```python
from build123d import *

# Parameters (mm, degrees)
SKETCH1_R           = 3
BOSS_EXTRUDE1_DEPTH = 6.35


with BuildPart() as part:
    # Sketch1 → Boss-Extrude1 (new body)
    with BuildSketch(Plane(origin=(0, 0, 0), x_dir=(1, 0, 0), z_dir=(0, 1, 0))):
        Polygon((0, 0), (63.3, 0), (63.3, 5), (69.65, 5), (69.65, 15), (63.3, 15), (63.3, 20), (0, 20), (0, 15), (-6.35, 15), (-6.35, 5), (0, 5), align=None)
        with Locations(Location((7.65, 10, 0), (0, 0, 270))):
            Circle(SKETCH1_R, mode=Mode.SUBTRACT)
        with Locations(Location((19.65, 10, 0), (0, 0, 270))):
            Circle(SKETCH1_R, mode=Mode.SUBTRACT)
        with Locations(Location((31.65, 10, 0), (0, 0, 270))):
            Circle(SKETCH1_R, mode=Mode.SUBTRACT)
        with Locations(Location((43.65, 10, 0), (0, 0, 270))):
            Circle(SKETCH1_R, mode=Mode.SUBTRACT)
        with Locations(Location((55.65, 10, 0), (0, 0, 270))):
            Circle(SKETCH1_R, mode=Mode.SUBTRACT)
    extrude(amount=BOSS_EXTRUDE1_DEPTH)


solid = part.part
```
CAD build for the part. Positions are in the model's coordinates, mm. A direction names the side the tool comes from. Coordinates: 2 decimals unless noted, no trailing zeros. Order: outer loops, then holes, each group sorted by start corner. A loop starts at its lowest first (then second) coordinate and runs counter-clockwise, first axis right, second up. Notation, with made-up numbers: (20, -23) - (41, -23) arc R25 cw to (41, -4) - close; hole circle Ø4 at (-25, 25). An arc over 180 degrees is marked (long way). Use a Markdown table: item, result. Add a question column.
(1) Drill centre lines: line 1 along X through (y, z) = (5.25, -10); line 2 along X through (y, z) = (3, -11.5); line 3 along X through (y, z) = (3, -17.75). Where is each one in solid material? Low to high. Write a range as [from, to].
(2) Saw through at A-A (z = -10). Give the cut face in (x, y), then the cut area to 3 significant figures.
(3) Pull direction X, two halves, no side cores. Call faces 4 (the face through (-6.35, 3, -10)), 5 (the face through (32, 3, -20)), 6 (the face through (16.72, 3.13, -10.65)): +X half, -X half, draft (parallel to the pull), parting line (faces both ways), or undercut.
(4) Saw through at B-B (y = 2.75). Give the cut face in (x, z), then the cut area to 3 significant figures.
(5) Which spindle directions (+Z, -Z, +X, -X, +Y, -Y) get a long thin tool onto all of the face, cutting with end or side? Do faces 1 (the face through (63.3, 3, -17)), 2 (the face through (0, 3, -18)), 3 (the face through (63.3, 3, -2)). Say none if no direction does.
(6) Saw through at D-D (z = -15.75). Give the cut face in (x, y), then the cut area to 3 significant figures.
(7) Flat gauge pins, fed straight in: pin 1 (3 mm diameter, centred on x = -2, y = 4.5, fed in from -Z); pin 2 (3 mm diameter, centred on x = -3, y = 4, fed in from +Z); pin 3 (1.5 mm diameter, centred on y = 2, z = -16.5, fed in from +X). Where does each tip first touch, or does it go through?
(8) Saw through at C-C (x = 55.65). Give the cut face in (y, z).
Solved:
| question | item | result |
|---|---|---|
| 1 | line 1 | x = [-6.35, 4.65], [10.65, 16.65], [22.65, 28.65], [34.65, 40.65], [46.65, 52.65], [58.65, 69.65] |
| 1 | line 2 | x = [-6.35, 5.05], [10.25, 17.05], [22.25, 29.05], [34.25, 41.05], [46.25, 53.05], [58.25, 69.65] |
| 1 | line 3 | x = [0, 63.3] |
| 2 | outline | (-6.35, 0) - (4.65, 0) - (4.65, 6.35) - (-6.35, 6.35) - close; (10.65, 0) - (16.65, 0) - (16.65, 6.35) - (10.65, 6.35) - close; (22.65, 0) - (28.65, 0) - (28.65, 6.35) - (22.65, 6.35) - close; (34.65, 0) - (40.65, 0) - (40.65, 6.35) - (34.65, 6.35) - close; (46.65, 0) - (52.65, 0) - (52.65, 6.35) - (46.65, 6.35) - close; (58.65, 0) - (69.65, 0) - (69.65, 6.35) - (58.65, 6.35) - close |
| 2 | area | 292 mm² |
| 3 | face 4 | -X half |
| 3 | face 5 | draft |
| 3 | face 6 | undercut |
| 4 | outline | (-6.35, -15) - (0, -15) - (0, -20) - (63.3, -20) - (63.3, -15) - (69.65, -15) - (69.65, -5) - (63.3, -5) - (63.3, 0) - (0, 0) - (0, -5) - (-6.35, -5) - close; hole circle Ø6 at (7.65, -10); hole circle Ø6 at (19.65, -10); hole circle Ø6 at (31.65, -10); hole circle Ø6 at (43.65, -10); hole circle Ø6 at (55.65, -10) |
| 4 | area | 1,250 mm² |
| 5 | face 1 | -Z, +X, +Y, -Y |
| 5 | face 2 | -Z, -X, +Y, -Y |
| 5 | face 3 | +Z, +X, +Y, -Y |
| 6 | outline | (0, 0) - (63.3, 0) - (63.3, 6.35) - (0, 6.35) - close |
| 6 | area | 402 mm² |
| 7 | pin 1 | stops at z = -15 |
| 7 | pin 2 | stops at z = -5 |
| 7 | pin 3 | stops at x = 63.3 |
| 8 | outline | (0, -20) - (6.35, -20) - (6.35, -13) - (0, -13) - close; (0, -7) - (6.35, -7) - (6.35, 0) - (0, 0) - close |
